Input: dimensioned drawing with shaded views. Units: mm. Origin: part minimum x, y, z. Coordinates: 2 decimals unless noted, no trailing zeros. Order: outer loops, then holes, each group sorted by start corner. A loop starts at its lowest first (then second) coordinate and runs counter-clockwise, first axis right, second up. Notation, with made-up numbers: M -21,45 L 6,45 A12 ccw 6,62 Z; hole C -10,11 d8. An arc over 180 degrees is marked long. Use CSV: the item, a comma, the result in double quotes. Start each with the question number.
1. First-contact query: P1, Ø2, axis at x = 5.01, y = 24, coming from the +Z side (1 decimal); P2, Ø1.6, axis at x = 29.01, y = 6, coming from the -Z side. Flat tips, straight axial feed; report the tip coordinate or a pass-through.
2. Material intervals for line 1 (Y direction, x = 30, z = 10.5) (1 decimal); line 2 (X direction, y = 24.75, z = 3) (1 decimal); line 3 (X direction, y = 5.5, z = 3.5), sorted ascending.
3. Section query A-A on z = 4. Return the cut outline in (x, y) (1 decimal), and give its area (3 significant figures).
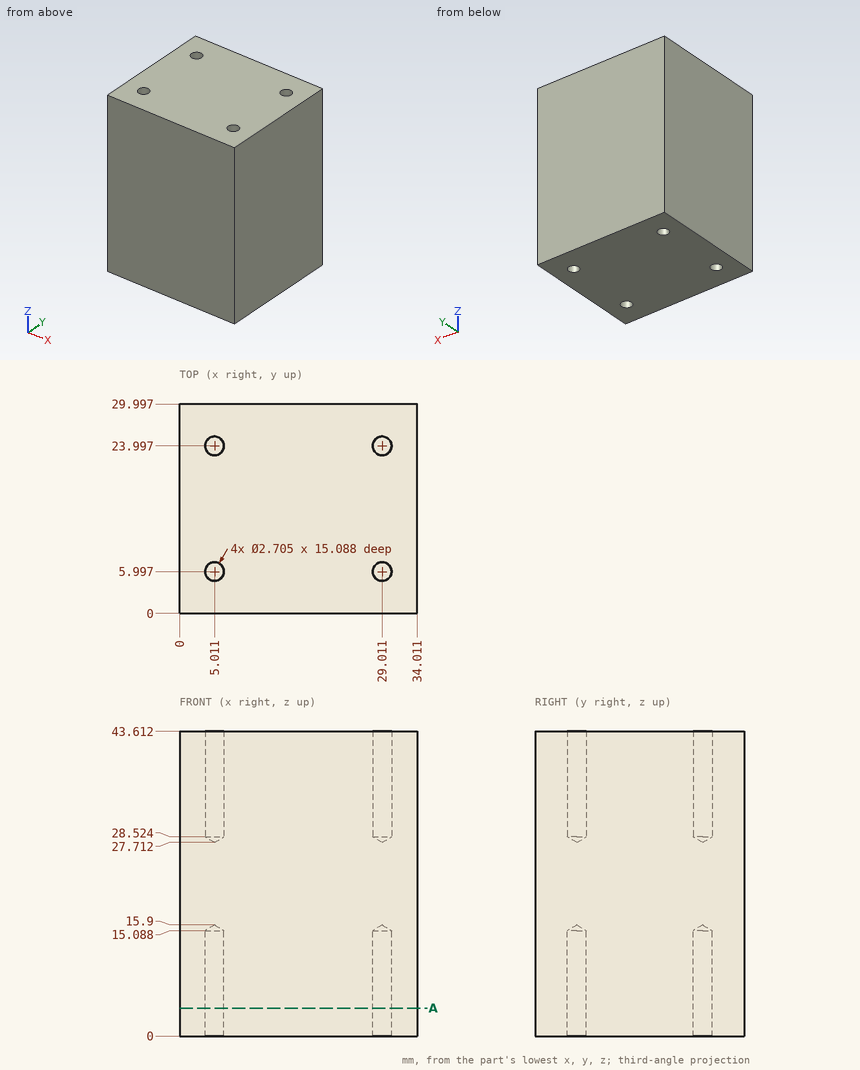
Results list:
1,P1,"stops at z = 28.3"
1,P2,"stops at z = 15.42"
2,line 1,"y = 0 to 5.1, 6.9 to 23.1, 24.9 to 30"
2,line 2,"x = 0 to 3.9, 6.1 to 27.9, 30.1 to 34"
2,line 3,"x = 0 to 3.75, 6.27 to 27.75, 30.27 to 34.01"
3,outline,"M 0,0 L 34,0 L 34,30 L 0,30 Z; hole C 5,6 d2.7; hole C 5,24 d2.7; hole C 29,6 d2.7; hole C 29,24 d2.7"
3,area,"997 mm²"
